Source: three-view drawing plus pictorial views. Frame: mm from the lowest corner of the part. Coordinates: 2 decimals unless noted, no trailing zeros. Write each loop counter-clockwise with the first axis right and the second up, starting at its lowest first coordinate (ties: lowest second). Pieces come first, ordered by that corner, then holes.
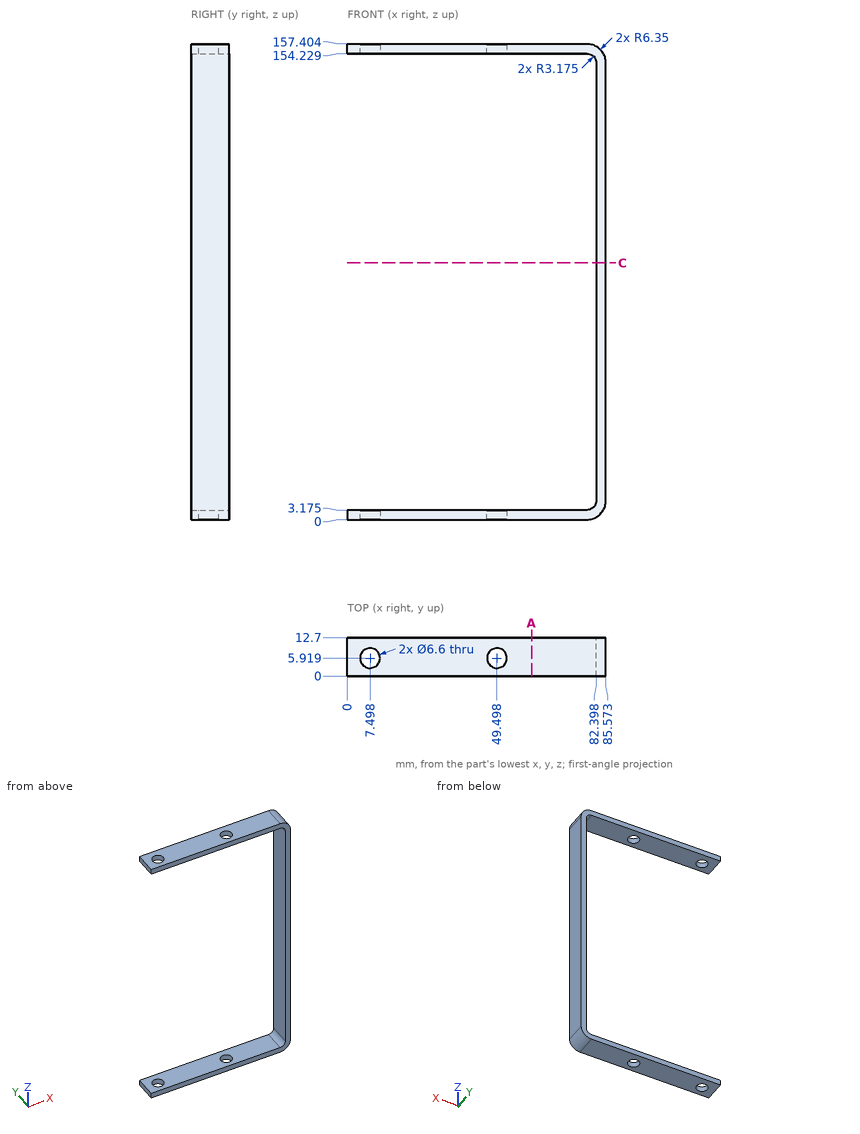
Item 1: Material intervals for line 1 (Z direction, x = 34, y = 8.75) (1 decimal); line 2 (X direction, y = 4.5, z = 60.5), sorted ascending.
Item 2: Section query A-A, the plane x = 61. Return loops of the section in (y, z) (1 decimal).
Item 3: Pin query (flat end, axial travel): pin 1 Ø4 at (x, y) = (49.5, 5.92) entering from +Z; pin 2 Ø4 at (y, z) = (3.5, 79.5) entering from -X. Return the tip coordinate at first contact, or that it passes through.
Item 4: Section query C-C, the plane z = 85. Return loops of the section in (x, y), then the cut area to 3 significant figures.
The answers:
1. line 1: z = 0 to 3.2, 154.2 to 157.4
1. line 2: x = 82.4 to 85.57
2. outline: (0, 0) - (12.7, 0) - (12.7, 3.2) - (0, 3.2) - close; (0, 154.2) - (12.7, 154.2) - (12.7, 157.4) - (0, 157.4) - close
3. pin 1: passes through
3. pin 2: stops at x = 82.4
4. outline: (82.4, 0) - (85.57, 0) - (85.57, 12.7) - (82.4, 12.7) - close
4. area: 40.3 mm2
